from build123d import *

# Parameters (mm, degrees)
F1_DEPTH = 7.62
F2_W     = 14.732
F2_H     = 14.732
F5_DEPTH = 25.4
F6_DEPTH = 25.4
F7_DEPTH = 25.4
F8_R     = 7.366
F9_DEPTH = 25.4
F10_T    = -0.254


with BuildPart() as f1:
    # F0 (on Front) → F1 (new body)
    with BuildSketch(Plane.XZ):
        with BuildLine():
            ThreePointArc((0, 5.08), (1.4878975516, 1.4878975516), (5.08, 0))
            Line((5.08, 0), (45.085, 0))
            ThreePointArc((45.085, 0), (48.6771024484, 1.4878975516), (50.165, 5.08))
            Line((50.165, 5.08), (50.165, 35.306))
            ThreePointArc((50.165, 35.306), (48.6771024484, 38.8981024484), (45.085, 40.386))
            Line((45.085, 40.386), (5.08, 40.386))
            ThreePointArc((5.08, 40.386), (1.4878975516, 38.8981024484), (0, 35.306))
            Line((0, 35.306), (0, 5.08))
        make_face()
    extrude(amount=F1_DEPTH)

    # F2 (on face) → F5 (cut)
    with BuildSketch(Plane.XZ.offset(7.62)):
        with Locations((37.719, 31.75)):
            Rectangle(F2_W, F2_H)
    extrude(amount=-F5_DEPTH, mode=Mode.SUBTRACT)

    # F3 (on face) → F6 (cut)
    with BuildSketch(Plane.XZ.offset(7.62)):
        Polygon((31.0508851266, 17.4752), (31.0508851266, 1.27), (45.085, 9.3726), align=None)
    extrude(amount=-F6_DEPTH, mode=Mode.SUBTRACT)

    # F4 (on face) → F7 (cut)
    with BuildSketch(Plane.XZ.offset(7.62)):
        Polygon((9.5977203913, 5.108581493), (12.3952, 1.27), (15.1585802409, 5.108581493), (19.6948698543, 6.5898499511), (16.8980608845, 10.4263776555), (16.8911139309, 15.1761725752), (12.3783031817, 13.7024369881), (7.8586276198, 15.1629618442), (7.8690663965, 10.4131733151), (5.08, 6.5684745393), align=None)
    extrude(amount=-F7_DEPTH, mode=Mode.SUBTRACT)

    # F8 (on face) → F9 (cut)
    with BuildSketch(Plane.XZ.offset(7.62)):
        with Locations((12.446, 31.75)):
            Circle(F8_R)
    extrude(amount=-F9_DEPTH, mode=Mode.SUBTRACT)

    # F10
    f10_openings = [f1.faces().sort_by_distance(p)[0] for p in [
        (24.768491, 0, 18.728729),
    ]]
    offset(amount=F10_T, openings=f10_openings, kind=Kind.INTERSECTION)


solid = f1.part
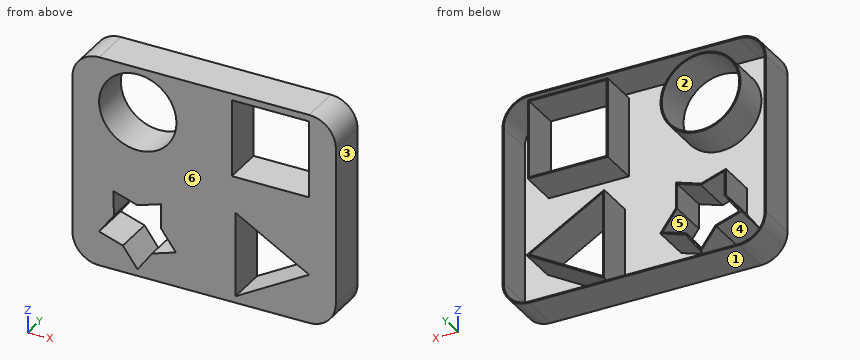
Could you check a few things on this model? Use its own coordinates, in mm. Face numbers are marked on the shaded views. A direction names the side the tool comes from. Give positions to 0.01 mm unless a question says otherwise; leave off trailing zeros. Order: outer loops, then holes, each group sorted by start corner. A loop starts at its lowest first (then second) coordinate and runs counter-clockwise, first axis right, second up.
1. For pin 1 (12 mm diameter, centred on x = 24, z = 18, fed in from +Y); pin 2 (13.5 mm diameter, centred on x = 12.446, z = 31.75, fed in from -Y), each with a flat end and sliding along its axis, tell me the tip position at first contact or that it passes through.
Answers below:
pin 1: stops at y = -7.37
pin 2: passes through
2. Suppose I cut it at B-B (y = -5.25). State how many separate pieces and enclosed holes the cut face has, plus the area to 3 significant figures.
Answers below:
separate pieces: 5
enclosed holes: 5
area: 95.9 mm2
3. Suppose I cut it at A-A (z = 31.75). Write out the boundary of the cut face in (x, y) (3 decimals).
Answers below:
outline: (0, -7.62) - (5.08, -7.62) - (5.08, 0) - (4.826, 0) - (4.826, -7.366) - (0.254, -7.366) - (0.254, 0) - (0, 0) - close; (19.812, -7.62) - (30.353, -7.62) - (30.353, 0) - (30.099, 0) - (30.099, -7.366) - (20.066, -7.366) - (20.066, 0) - (19.812, 0) - close; (45.085, -7.62) - (50.165, -7.62) - (50.165, 0) - (49.911, 0) - (49.911, -7.366) - (45.339, -7.366) - (45.339, 0) - (45.085, 0) - close
4. Which directions (+Z, -Z, +X, -X, +Y, -Y) give clear straight access to the entire face, cutting with the end or side of a thin tool? Please do the marked faces 4, 5 and 6.
Answers below:
face 4: +Y
face 5: +Y, -Y
face 6: +Z, -Z, +X, -X, -Y
5. Suppose I cut it at C-C (x = 40.5). Write out the boundary of the cut face in (y, z).
Answers below:
outline: (-7.62, 0) - (0, 0) - (0, 0.25) - (-7.37, 0.25) - (-7.37, 6.43) - (0, 6.43) - (0, 6.73) - (-7.62, 6.73) - close; (-7.62, 12.02) - (0, 12.02) - (0, 12.31) - (-7.37, 12.31) - (-7.37, 24.13) - (0, 24.13) - (0, 24.38) - (-7.62, 24.38) - close; (-7.62, 39.12) - (0, 39.12) - (0, 39.37) - (-7.37, 39.37) - (-7.37, 40.13) - (0, 40.13) - (0, 40.39) - (-7.62, 40.39) - close
6. Thinking about a two-plate mould opening in Z: for the marked faces 1, 2 and 3, which applies, +Z half, -Z half, draft (parallel to the pull), parting line (faces both ways), or undercut?
Answers below:
face 1: -Z half
face 2: undercut
face 3: draft
7. I need wall thicknesses on L1, parallel to Z at x = 29.5, y = -3; L2, parallel to Z at x = 11, y = -4.5; L3, parallel to Z at x = 34, y = -3. Which ranges of each line are inside material? Lowest first, please.
Answers below:
L1: z = 0 to 0.25, 40.13 to 40.39
L2: z = 0 to 0.25, 2.75 to 3.18, 14.15 to 14.41, 24.27 to 24.53, 38.97 to 39.23, 40.13 to 40.39
L3: z = 0 to 0.25, 2.68 to 2.97, 15.77 to 16.07, 24.13 to 24.38, 39.12 to 39.37, 40.13 to 40.39
8. Suppose I cut it at D-D (z = 18.5). Write out the boundary of the cut face in (x, y) (3 decimals), plus the area to 3 significant figures.
Answers below:
outline: (0, -7.62) - (50.165, -7.62) - (50.165, 0) - (49.911, 0) - (49.911, -7.366) - (0.254, -7.366) - (0.254, 0) - (0, 0) - close
area: 16.5 mm2
